Source: CAD feature listing. Evaluate the final solid. Frame: model axes, mm. Give positions to 0.01 mm unless a question says otherwise; leave off trailing zeros. Write each loop counter-clockwise with the first axis right and the second up, starting at its lowest first coordinate (ties: lowest second). Pieces come first, ordered by that corner, then holes. Notation, with made-up numbers: M 32,22 L 47,22 A11 ccw 47,40 Z; hole C 14.5,-2 d10. An arc over 180 degrees is marked long. Return JSON: item names as keys, results as strings.
```python
from build123d import *

# Parameters (mm, degrees)
EXTRUDE1_DEPTH = 47.625
FILLET1_R      = 0.635


with BuildPart() as part:
    # Sketch2 → Extrude1 (new, symmetric)
    with BuildSketch(Plane(origin=(0, 0, 0), x_dir=(0, 0, -1), z_dir=(1, 0, 0))):
        with BuildLine():
            Line((-14.2875, 3.175), (-2.778125, 3.175))
            ThreePointArc((-2.778125, 3.175), (0, 1.5748), (2.778125, 3.175))
            Line((2.778125, 3.175), (14.2875, 3.175))
            Line((14.2875, 3.175), (14.2875, 0))
            Line((14.2875, 0), (-14.2875, 0))
            Line((-14.2875, 0), (-14.2875, 3.175))
        make_face()
    extrude(amount=EXTRUDE1_DEPTH, both=True)

    # Fillet1
    fillet1_edges = [part.edges().sort_by_distance(p)[0] for p in [
        (0, 3.175, 14.2875),
        (0, 3.175, -14.2875),
        (0, 0, -14.2875),
        (0, 0, 14.2875),
    ]]
    fillet(fillet1_edges, radius=FILLET1_R)


solid = part.part
```
1) Line query: line 1 (Z direction, x = -25, y = 2.7); line 2 (Z direction, x = -24, y = 2.4); line 3 (Z direction, x = -12, y = 0.45). Output: solid intervals per line, ascending. Write a range as [from, to].
Numbers:
{"line 1": "z = [-14.27, -2.44], [2.44, 14.27]", "line 2": "z = [-14.29, -2.15], [2.15, 14.29]", "line 3": "z = [-14.26, 14.26]"}
2) Cut plane B-B, the plane z = 1.75. Return the cut outline in (x, y) (3 decimals), then the cut area to 3 significant figures.
Numbers:
{"outline": "M -47.625,0 L 47.625,0 L 47.625,2.093 L -47.625,2.093 Z", "area": "199 mm²"}
3) Draft query along Z for faces 1 (the face through (-47.625, 1, 0)), 2 (the face through (1, 2, 14.288)), 3 (the face through (0.667, 1.575, 0.047)). Return one class per face: released by +Z, released by -Z, zero draft, split by the parting line, or undercut.
Numbers:
{"face 1": "zero draft", "face 2": "released by +Z", "face 3": "undercut"}
4) Cut plane A-A, the plane x = -11. Return the cut outline in (y, z) (1 decimal), then the cut area to 3 significant figures.
Numbers:
{"outline": "M 0,-13.7 A0.6 ccw 0.6,-14.3 L 2.5,-14.3 A0.6 ccw 3.2,-13.7 L 3.2,-2.8 A3.2 cw 3.2,2.8 L 3.2,13.7 A0.6 ccw 2.5,14.3 L 0.6,14.3 A0.6 ccw 0,13.7 Z", "area": "84.1 mm²"}
